The listing builds one solid part. Answer for the finished solid, in the listing's coordinates (mm). A direction names the side the tool comes from. Round coordinates to 2 decimals unless told otherwise and drop trailing zeros. Order: outer loops, then holes, each group sorted by start corner. A loop starts at its lowest first (then second) coordinate and runs counter-clockwise, first axis right, second up. Notation, with made-up numbers: M 46.5,16.25 L 89.5,16.25 A24 cw 89.5,49.25 Z; hole C 24,-37.5 d6. An arc over 180 degrees is marked long. Put each result on its own line as item: value. Start each with the question number.
1. Each of these flat-tipped pins is pushed along its axis until it touches: pin 1 Ø4 at (x, z) = (-354, 0) entering from +Y; pin 2 Ø2 at (x, z) = (-340, 2) entering from +Y; pin 3 Ø1 at (y, z) = (-41.5, 2) entering from -X. Where does it stop, or does it pass through?
2. Consider line 1 (Y direction, x = -330.2, z = 0.1); line 2 (X direction, y = 0, z = -0.35); line 3 (X direction, y = -0.5, z = -2.75). Determine where each line is inside the solid, lowest interval first.
3. The part is cut by section A-A (y = 0). Give the vertices of the cut face in (x, z), then the cut area to 3 significant figures.
4. The part is cut by section B-B (x = -88.5). Give the vertices of the cut face in (y, z), then the cut area to 3 significant figures.
5. The mould has two halves that part along Z. Classify faces 5 (the face through (-398.227, -1.618, -2.785)), 6 (the face through (-396.983, -1.588, -0.022)), 7 (the face through (21.586, -0.436, 0.022)): +Z half, -Z half, draft (parallel to the pull), parting line (faces both ways), or undercut.
6. Which of the six approach directions +Z, -Z, +X, -X, +Y, -Y give full straight-line access (tool end or side, diameter ignored) to faces 1 (the face through (24.887, 0.503, -0.022)), 2 (the face through (-161.555, 45.767, 0.022)), 3 (the face through (20.34, -0.41, -2.75)), 4 (the face through (-157.43, -41.91, -0.02))?
Autodesk Inventor part; units mm, degrees
ref_plane "YZ Plane" through (0, 0, 0) normal (1, 0, 0) x (0, 1, 0)
ref_plane "XZ Plane" through (0, 0, 0) normal (0, 1, 0) x (-1, 0, 0)
ref_plane "XY Plane" through (0, 0, 0) normal (0, 0, 1) x (1, 0, 0)
sketch "Sketch2" plane through (0, 0, 0) normal (0, 0, 1) x (1, 0, 0)
  arc A0 (2.7403, -21.4154) -> (2.7403, 21.4154) centre (0, 0) ccw
  arc A1 (-322.1404, 62.9864) -> (-322.1404, -62.9864) centre (-330.2, 0) ccw
  line L0 (-322.1404, 62.9864) -> (2.7403, 21.4154)
  line L1 (2.7403, -21.4154) -> (-322.1404, -62.9864)
  dimension "d1" = 330.2
  dimension "d3" = 43.18
  dimension "d4" = 127
sketch "Sketch3" plane through (0, 0, 0) normal (0, 1, 0) x (-1, 0, 0)
  line L0 (-2.7403, 0) -> (-21.59, 0)
  line L1 (-26.1366, 3.9497) -> (-20.3454, 3.9497)
  line L2 (-20.3454, 3.9497) -> (-20.3454, 1.5875)
  line L3 (-20.3454, 1.5875) -> (-21.59, 1.5875)
  line L4 (-21.59, 1.5875) -> (-21.59, -1.5875)
  line L5 (-21.59, -1.5875) -> (-20.3454, -1.5875)
  line L6 (-20.3454, -1.5875) -> (-20.3454, -3.9497)
  line L7 (-20.3454, -3.9497) -> (-26.1366, -3.9497)
  line L8 (-26.1366, -3.9497) -> (-26.1366, -1.5875)
  line L9 (-26.1366, -1.5875) -> (-24.892, -1.5875)
  line L10 (-24.892, -1.5875) -> (-24.892, 1.5875)
  line L11 (-24.892, 1.5875) -> (-26.1366, 1.5875)
  line L12 (-26.1366, 3.9497) -> (-26.1366, 1.5875)
  point P0 (0, 0)
  point P1 (-24.892, 0)
  dimension "d8" = 5.7912
  dimension "d9" = 7.8994
  dimension "d10" = 3.175
  dimension "d11" = 3.302
sweep "Sweep1" add profiles "Sketch3" path "Sketch2"
properties part number "IntakeChain" material "Steel"
Resolved:
1. pin 1: y = 64.19
1. pin 2: y = 67.48
1. pin 3: x = -384.51
2. line 1: -66.8 to -63.5, 63.5 to 66.8
2. line 2: -397 to -393.7, 21.59 to 24.89
2. line 3: -398.24 to -392.45, 20.34 to 26.13
3. outline: M -398.25,-3.95 L -392.46,-3.95 L -392.46,-1.59 L -393.7,-1.59 L -393.7,1.59 L -392.46,1.59 L -392.46,3.95 L -398.25,3.95 L -398.25,1.59 L -397,1.59 L -397,-1.59 L -398.25,-1.59 Z; M 20.35,-3.95 L 26.14,-3.95 L 26.14,-1.59 L 24.89,-1.59 L 24.89,1.59 L 26.14,1.59 L 26.14,3.95 L 20.35,3.95 L 20.35,1.59 L 21.59,1.59 L 21.59,-1.59 L 20.35,-1.59 Z
3. area: 75.7 mm2
4. outline: M -37.67,-3.95 L -31.84,-3.95 L -31.84,-1.59 L -33.09,-1.59 L -33.09,1.59 L -31.84,1.59 L -31.84,3.95 L -37.67,3.95 L -37.67,1.59 L -36.42,1.59 L -36.42,-1.59 L -37.67,-1.59 Z; M 31.84,-3.95 L 37.67,-3.95 L 37.67,-1.59 L 36.42,-1.59 L 36.42,1.59 L 37.67,1.59 L 37.67,3.95 L 31.84,3.95 L 31.84,1.59 L 33.09,1.59 L 33.09,-1.59 L 31.84,-1.59 Z
4. area: 76.3 mm2
5. face 5: draft
5. face 6: undercut
5. face 7: undercut
6. face 1: +X
6. face 2: +X, +Y
6. face 3: +Z, -Z
6. face 4: none
